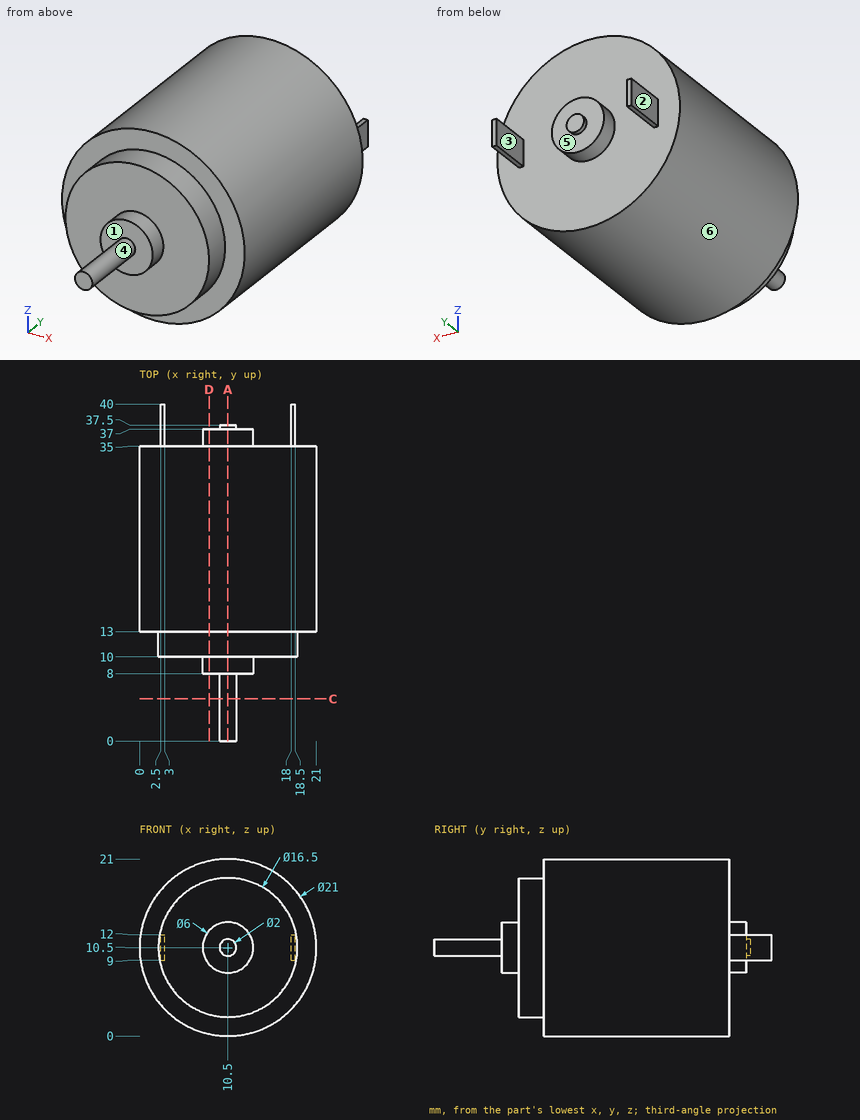
Part print with two shaded views. Sizes in mm from the minimum x, y, z corner. A direction names the side the tool comes from. Coordinates: 2 decimals unless noted, no trailing zeros. Write each loop counter-clockwise with the first axis right and the second up, starting at its lowest first coordinate (ties: lowest second). Pieces come first, ordered by that corner, then holes. Notation, with made-up numbers: (-7.5, 6.25) - (40.5, 6.25) arc R17 cw to (40.5, 14.25) - close; hole circle Ø2 at (75.5, 52). An arc over 180 degrees is marked (long way). One line per item, written item: value. Start each with the question number.
1. Slice it at C-C (y = 5). Write the cut outline in (x, z).
2. Slice it at D-D (x = 8.25). Write the cut outline in (y, z), plus the area to 3 significant figures.
3. Tool access for the marked faces 4, 5 and 6: list every direction of +Z, -Z, +X, -X, +Y, -Y with a clear straight run to the whole face (end or side of a thin tool).
4. Slice it at A-A (x = 10.5). Write the cut outline in (y, z), plus the area to 4 significant figures.
5. Probe line 1 (Y direction, x = 18, z = 3.75); line 2 (Y direction, x = 14.5, z = 11.25); line 3 (X direction, y = 15.5, z = 17). List the from-to ranges inside material, lowest first. Write a range as from..to.
6. Mould opens along X. For the marked faces 1, 2 and 3 say: released by +X, released by -X, zero draft, split by the parting line, or undercut.
7. Flat gauge pins, fed straight in: pin 1 (1.5 mm diameter, centred on x = 6.5, y = 16.5, fed in from +Z); pin 2 (2 mm diameter, centred on x = 10, z = 11, fed in from +Y); pin 3 (1 mm diameter, centred on x = 12.5, y = 18.5, fed in from -Z). Where does each tip first touch, or does it go through?
Answers below:
1. outline: circle Ø2 at (10.5, 10.5)
2. outline: (8, 8.52) - (10, 8.52) - (10, 2.56) - (13, 2.56) - (13, 0.24) - (35, 0.24) - (35, 8.52) - (37, 8.52) - (37, 12.48) - (35, 12.48) - (35, 20.76) - (13, 20.76) - (13, 18.44) - (10, 18.44) - (10, 12.48) - (8, 12.48) - close
2. area: 515 mm^2
3. face 4: -Y
3. face 5: +Y
3. face 6: +Y, -Y
4. outline: (0, 9.5) - (8, 9.5) - (8, 7.5) - (10, 7.5) - (10, 2.25) - (13, 2.25) - (13, 0) - (35, 0) - (35, 7.5) - (37, 7.5) - (37, 9.5) - (37.5, 9.5) - (37.5, 11.5) - (37, 11.5) - (37, 13.5) - (35, 13.5) - (35, 21) - (13, 21) - (13, 18.75) - (10, 18.75) - (10, 13.5) - (8, 13.5) - (8, 11.5) - (0, 11.5) - close
4. area: 552.5 mm^2
5. line 1: y = 13..35
5. line 2: y = 10..35
5. line 3: x = 2.25..18.75
6. face 1: zero draft
6. face 2: released by -X
6. face 3: undercut
7. pin 1: stops at z = 20.48
7. pin 2: stops at y = 37.5
7. pin 3: stops at z = 0.11
